from build123d import *

# Parameters (mm, degrees)
PAD_DEPTH     = 800
SKETCH001_W   = 48.320911
SKETCH001_H   = 733.872097
SKETCH001_W_2 = 18.120416
SKETCH001_H_2 = 694.611473
PAD001_DEPTH  = 15


with BuildPart() as part:
    # Sketch → Pad (new body)
    with BuildSketch(Plane.YZ):
        Polygon((-49.460372, 70.261276), (45.539628, 70.261276), (45.539628, -59.738724), (-49.460372, -59.738724), (-49.460372, -64.738724), (50.539628, -64.738724), (50.539628, 75.261276), (-49.460372, 75.261276), align=None)
    extrude(amount=PAD_DEPTH)

    # Sketch001 → Pad001 (join)
    with BuildSketch(Plane.ZX.offset(50.539628)):
        with Locations((2.740473, 401.065539)):
            Rectangle(SKETCH001_W, SKETCH001_H)
        with Locations((1.733778, 404.588916)):
            Rectangle(SKETCH001_W_2, SKETCH001_H_2, mode=Mode.SUBTRACT)
    extrude(amount=PAD001_DEPTH)


solid = part.part
Source: CAD feature listing. Evaluate the final solid. Frame: model axes, mm. A direction names the side the tool comes from. Give positions to 0.01 mm unless a question says otherwise; leave off trailing zeros. Order: outer loops, then holes, each group sorted by start corner. A loop starts at its lowest first (then second) coordinate and runs counter-clockwise, first axis right, second up. Notation, with made-up numbers: (57.5, 6) -> (110.5, 6) arc R34 ccw to (110.5, 41) -> close; hole circle Ø8 at (-31, -13). An arc over 180 degrees is marked (long way). Write item = value, one per line.
Q1. Cut plane A-A, the plane y = 4. Output: boundary loops of the cut face in (x, z), and give its area (3 significant figures).
Data:
outline = (0, -64.74) -> (800, -64.74) -> (800, -59.74) -> (0, -59.74) -> close; (0, 70.26) -> (800, 70.26) -> (800, 75.26) -> (0, 75.26) -> close
area = 8,000 mm^2
Q2. Pull-direction query (X, two-part tool) for faces 1 (the face through (800, 48, 6)), 2 (the face through (406, 65.54, 13)), 3 (the face through (400, 50.54, 2)); classes: released by +X, released by -X, zero draft, split by the parting line, or undercut.
Data:
face_1 = released by +X
face_2 = zero draft
face_3 = undercut
Q3. Cut plane B-B, the plane x = 346. Output: boundary loops of the cut face in (y, z).
Data:
outline = (-49.46, -64.74) -> (50.54, -64.74) -> (50.54, -21.42) -> (65.54, -21.42) -> (65.54, -7.33) -> (50.54, -7.33) -> (50.54, 10.79) -> (65.54, 10.79) -> (65.54, 26.9) -> (50.54, 26.9) -> (50.54, 75.26) -> (-49.46, 75.26) -> (-49.46, 70.26) -> (45.54, 70.26) -> (45.54, -59.74) -> (-49.46, -59.74) -> close
Q4. Pin query (flat end, axial travel): pin 1 (7.5 mm diameter, centred on x = 238.5, y = 60, fed in from -Z); pin 2 (9 mm diameter, centred on x = 410, z = -1, fed in from +Y); pin 3 (12 mm diameter, centred on y = 58, z = -2, fed in from +X). Return the tip coordinate at first contact, or that it passes through.
Data:
pin_1 = -21.42
pin_2 = 50.54
pin_3 = 768
Q5. Cut plane C-C, the plane z = -33.5. Output: boundary loops of the cut face in (x, y), and give its area (3 significant figures).
Data:
outline = (0, 45.54) -> (800, 45.54) -> (800, 50.54) -> (0, 50.54) -> close
area = 4,000 mm^2
Q6. Set-up query: faces 4 (the face through (34.129, 58, 2)), 5 (the face through (396, 58, -21.42)), 6 (the face through (768.002, 58, 2)). Return all of +Z, -Z, +X, -X, +Y, -Y with unobstructed straight access to the full face (end or side cutting, diameter ignored); none if empty.
Data:
face_4 = +Z, -Z, -X, +Y
face_5 = -Z, +X, -X, +Y
face_6 = +Z, -Z, +X, +Y
Q7. Material intervals for line 1 (Z direction, x = 432.5, y = 21); line 2 (X direction, y = 52, z = 2.5); line 3 (Y direction, x = 52, z = -3.5), sorted ascending. Write a range as from..to.
Data:
line_1 = -64.74..-59.74, 70.26..75.26
line_2 = 34.13..57.28, 751.89..768
line_3 = 45.54..65.54
